```python
from build123d import *

# Parameters (mm, degrees)
F0_W     = 1000
F0_H     = 1710
F1_DEPTH = 40
F0_W_2   = 30
F0_H_2   = 30
F0_W_3   = 936
F0_H_3   = 1646
F2_DEPTH = 2


with BuildPart() as f1:
    # F0 (on Front) → F1 (new body)
    with BuildSketch(Plane.XZ):
        with Locations((459.7794299543, -895)):
            Rectangle(F0_W, F0_H)
        Polygon((-38.2205700457, -72), (-38.2205700457, -42), (-8.2205700457, -42), (927.7794299543, -42), (957.7794299543, -42), (957.7794299543, -72), (957.7794299543, -1718), (957.7794299543, -1748), (927.7794299543, -1748), (-8.2205700457, -1748), (-38.2205700457, -1748), (-38.2205700457, -1718), align=None, mode=Mode.SUBTRACT)
    extrude(amount=F1_DEPTH)

    # F0 (on Front) → F2 (join)
    with BuildSketch(Plane.XZ):
        with Locations((942.7794299543, -57)):
            Rectangle(F0_W_2, F0_H_2)
        with Locations((459.7794299543, -57)):
            Rectangle(F0_W_3, F0_H_2)
        with Locations((942.7794299543, -895)):
            Rectangle(F0_W_2, F0_H_3)
        with Locations((-23.2205700457, -57)):
            Rectangle(F0_W_2, F0_H_2)
        with Locations((-23.2205700457, -895)):
            Rectangle(F0_W_2, F0_H_3)
        with Locations((-23.2205700457, -1733)):
            Rectangle(F0_W_2, F0_H_2)
        with Locations((459.7794299543, -1733)):
            Rectangle(F0_W_3, F0_H_2)
        with Locations((942.7794299543, -1733)):
            Rectangle(F0_W_2, F0_H_2)
    extrude(amount=F2_DEPTH)


solid = f1.part
```
Design review of the part built by this model. Coordinates are the model's own, in mm. A direction names the side the tool comes from. Round coordinates to 2 decimals unless told otherwise and drop trailing zeros. Write each loop counter-clockwise with the first axis right and the second up, starting at its lowest first coordinate (ties: lowest second). Pieces come first, ordered by that corner, then holes.
Item 1: For faces 5 (the flat face through (453, -20, -40)), 6 (the flat face through (-38.221, -21, -907)), list the 3-axis set-ups (+Z, -Z, +X, -X, +Y, -Y) from which the entire face can be reached by the end or side of a thin tool; tool diameter is ignored.
Item 2: We need section A-A on z = -1224.5. Write out the cut boundary in (x, y), and give its area (3 significant figures).
Item 3: For probe 1 along X at (y, z) = (-32.5, -957); probe 2 along Z at (x, y) = (565, -30.5), list the stretches that pass through material, from the lowest coordinate up.
Item 4: We need section C-C on y = -21. Write out the cut boundary in (x, z).
Item 5: The part is to be moulded in two halves that separate along X. For faces 1 (the flat face through (-40.221, -20, -907)), 2 (the flat face through (937, -2, -638)), 3 (the flat face through (957.779, -21, -883)), 4 (the flat face through (453, -20, -1750)), say which applies: +X half, -X half, draft (parallel to the pull), parting line (faces both ways), or undercut.
Item 6: We need section B-B on x = 165. Write out the cut boundary in (y, z), and give its area (3 significant figures).
Returned:
1. face 5: +Z, +X, -X, +Y, -Y
1. face 6: -Y
2. outline: (-40.22, -40) - (-38.22, -40) - (-38.22, -2) - (-8.22, -2) - (-8.22, 0) - (-40.22, 0) - close; (927.78, -2) - (957.78, -2) - (957.78, -40) - (959.78, -40) - (959.78, 0) - (927.78, 0) - close
2. area: 280 mm2
3. probe 1: x = -40.22 to -38.22, 957.78 to 959.78
3. probe 2: z = -1750 to -1748, -42 to -40
4. outline: (-40.22, -1750) - (959.78, -1750) - (959.78, -40) - (-40.22, -40) - close; hole (-38.22, -1748) - (957.78, -1748) - (957.78, -42) - (-38.22, -42) - close
5. face 1: -X half
5. face 2: undercut
5. face 3: undercut
5. face 4: draft
6. outline: (-40, -1750) - (0, -1750) - (0, -1718) - (-2, -1718) - (-2, -1748) - (-40, -1748) - close; (-40, -42) - (-2, -42) - (-2, -72) - (0, -72) - (0, -40) - (-40, -40) - close
6. area: 280 mm2
